```python
from build123d import *

# Parameters (mm, degrees)
BOSS_EXTRUDE2_DEPTH = 2
BOSS_EXTRUDE3_DEPTH = 2
BOSS_EXTRUDE4_DEPTH = 2
FILLET1_R           = 1
FILLET2_R           = 1


with BuildPart() as part:
    # Sketch1 → Boss-Extrude2 (new body)
    with BuildSketch(Plane(origin=(0, 0, 0), x_dir=(1, 0, 0), z_dir=(0, 1, 0))):
        with BuildLine():
            Line((0, 0), (40, 0))
            Line((40, 0), (40, 7))
            ThreePointArc((40, 7), (39.121320344, 9.121320344), (37, 10))
            Line((37, 10), (3, 10))
            ThreePointArc((3, 10), (0.878679656, 9.121320344), (0, 7))
            Line((0, 7), (0, 0))
        make_face()
        with BuildLine():
            Line((4, 8), (36, 8))
            ThreePointArc((36, 8), (38, 6), (36, 4))
            Line((36, 4), (4, 4))
            ThreePointArc((4, 4), (2, 6), (4, 8))
        make_face(mode=Mode.SUBTRACT)
    extrude(amount=BOSS_EXTRUDE2_DEPTH)

    # Sketch2 → Boss-Extrude3 (add)
    with BuildSketch(Plane.XY):
        Polygon((0, 2), (-2.588190451, 11.659258263), (32.0528257, 31.659258263), (40, 2), align=None)
    extrude(amount=-BOSS_EXTRUDE3_DEPTH)

    # Sketch3 → Boss-Extrude4 (add)
    with BuildSketch(Plane(origin=(-5.695654535, 9.865163037, 0), x_dir=(0.866025403784438, 0.5000000000000012, 0), z_dir=(-0.5000000000000012, 0.866025403784438, 0))):
        with BuildLine():
            Line((3.588190451, 0), (43.588190451, 0))
            Line((43.588190451, 0), (43.588190451, 7))
            ThreePointArc((43.588190451, 7), (42.709510795, 9.121320344), (40.588190451, 10))
            Line((40.588190451, 10), (6.588190451, 10))
            ThreePointArc((6.588190451, 10), (4.466870107, 9.121320344), (3.588190451, 7))
            Line((3.588190451, 7), (3.588190451, 0))
        make_face()
        with BuildLine():
            Line((7.588190451, 4), (39.588190451, 4))
            ThreePointArc((39.588190451, 4), (41.588190451, 6), (39.588190451, 8))
            Line((39.588190451, 8), (7.588190451, 8))
            ThreePointArc((7.588190451, 8), (5.588190451, 6), (7.588190451, 4))
        make_face(mode=Mode.SUBTRACT)
    extrude(amount=BOSS_EXTRUDE4_DEPTH)

    # Fillet1
    fillet1_edges = [part.edges().sort_by_distance(p)[0] for p in [
        (20, 0, 0),
    ]]
    fillet(fillet1_edges, radius=FILLET1_R)

    # Fillet2
    fillet2_edges = [part.edges().sort_by_distance(p)[0] for p in [
        (13.732317625, 23.39130907, 0),
    ]]
    fillet(fillet2_edges, radius=FILLET2_R)


solid = part.part
```
Work out the finished part from the listing and answer in its coordinate system (mm). A direction names the side the tool comes from. Coordinates: 2 decimals unless noted, no trailing zeros. Order: outer loops, then holes, each group sorted by start corner. A loop starts at its lowest first (then second) coordinate and runs counter-clockwise, first axis right, second up. Notation, with made-up numbers: (49, 17) - (61, 17) arc R13 cw to (61, 25) - close; hole circle Ø1 at (69, 79.5). An arc over 180 degrees is marked (long way). Answer as a JSON object with one key per item and string values.
1. Consider line 1 (Z direction, x = 8.5, y = 4); line 2 (Y direction, x = 20, z = -9); line 3 (Y direction, x = 36, z = -8.5). Determine where each line is inside the solid, lowest interval first.
Output values:
{"line 1": "z = -2 to 0", "line 2": "y = 0 to 2, 24.7 to 27.01", "line 3": "y = 0 to 2"}
2. Find section A-A on z = -6.25. Determine the outline of the cut face in (x, y), plus the area to 3 significant figures.
Output values:
{"outline": "(-3.59, 13.39) - (-2.59, 11.66) - (-0.84, 12.67) - (-1.84, 14.4) - close; (0, 0) - (2.02, 0) - (2.02, 2) - (0, 2) - close; (29.31, 32.38) - (30.31, 30.65) - (32.05, 31.66) - (31.05, 33.39) - close; (37.98, 0) - (40, 0) - (40, 2) - (37.98, 2) - close", "area": "16.1 mm²"}
3. The mould has two halves that part along X. Classify faces 1 (the face through (19, 11, 0)), 2 (the face through (20, 1, -4)), 3 (the face through (35.97, 17.04, -0.99)), 4 (the face through (14.125, 23.271, -0.285)): +X half, -X half, draft (parallel to the pull), parting line (faces both ways), or undercut.
Output values:
{"face 1": "draft", "face 2": "undercut", "face 3": "+X half", "face 4": "-X half"}
4. A tool of negligible diameter and unlimited length cuts with its end or side. For faces 5 (the face through (-1.349, 13.513, -6.044)), 6 (the face through (2, 1, -6)), 7 (the face through (14.49, 21.52, -8.72)), from which of +Z, -Z, +X, -X, +Y, -Y can it reach the whole face along a straight path? Write none if from no direction.
Output values:
{"face 5": "+X, +Y", "face 6": "+Y, -Y", "face 7": "-Z, +X"}
5. Find section C-C on y = 4.5. Determine the outline of the cut face in (x, z).
Output values:
{"outline": "(-0.67, -2) - (39.33, -2) - (39.33, 0) - (-0.67, 0) - close"}
6. Each of these flat-tipped pins is pushed along its axis until it touches: P1, Ø15, axis at x = 21.5, y = 13, coming from the -Z side; P2, Ø4, axis at y = 28, z = -7, coming from the -X side; P3, Ø4, axis at x = 11, z = -7.5, coming from the +Y side. Where does it stop, or does it pass through?
Output values:
{"P1": "stops at z = -2", "P2": "stops at x = 18.71", "P3": "stops at y = 22.93"}
7. Find section B-B on x = 25. Count the separate pieces of the cut face and the enclosed holes in it, plus the area to 3 significant figures.
Output values:
{"separate pieces": "3", "enclosed holes": "0", "area": "76.6 mm²"}
